Build history of the part. All positions in model axes, mm. A direction names the side the tool comes from. Coordinates: 2 decimals unless noted, no trailing zeros. Write each loop counter-clockwise with the first axis right and the second up, starting at its lowest first coordinate (ties: lowest second). Pieces come first, ordered by that corner, then holes. Notation, with made-up numbers: (-35.5, 38.5) -> (13.5, 38.5) arc R9 ccw to (13.5, 49.5) -> close; hole circle Ø3 at (15.25, 28.25). An arc over 180 degrees is marked (long way). Write each question's results on one line, items separated by ' | '. Start each with the question number.
Q1. Saw through at A-A on z = 159.5. Give the cut face in (x, y).
Q2. Drill centre lines: line 1 (X direction, y = -4.75, z = 64); line 2 (X direction, y = -1.5, z = 0) (3 decimals); line 3 (X direction, y = -3.75, z = 58). Where is each one in solid material? Low to high.
Q3. Drop flat-ended pins along their axis: pin 1 Ø2.5 at (x, z) = (-20.32, 196.85) entering from +Y; pin 2 Ø2 at (x, y) = (-15, -4.5) entering from +Z. Give the stop position or say it passes through.
Q4. Tool access for faces 1 (the face through (-15.24, -3, 54)), 2 (the face through (-17, -6.35, 107)): list every direction of +Z, -Z, +X, -X, +Y, -Y with a clear straight run to the whole face (end or side of a thin tool).
Q5. Saw through at C-C on z = 85. Give the cut face in (x, y), and give its area (3 significant figures).
Q6. Saw through at B-B on y = -1.75. Count the separate pieces of the cut face and the enclosed holes in it, and give its area (3 significant figures).
Q7. Two-plate mould, pull along Z, no slides. Class faces 3 (the face through (6.92, -3.13, 153.79)), 4 (the face through (2.115, -3.131, 195.809)), 5 (the face through (25.4, -3, 102)): released by +Z, released by -Z, zero draft, split by the parting line, or undercut.
from build123d import *

# Parameters (mm, degrees)
SKETCH1_R           = 3.96875
SKETCH1_R_2         = 15.08125
SKETCH1_R_3         = 1.5875
BOSS_EXTRUDE1_DEPTH = 6.35


with BuildPart() as part:
    # Sketch1 → Boss-Extrude1 (new body)
    with BuildSketch(Plane(origin=(0, 0, 0), x_dir=(1, 0, 0), z_dir=(0, 1, 0))):
        with BuildLine():
            Line((25.4, -39.926769414), (25.4, -166.672190904))
            ThreePointArc((25.4, -166.672190904), (25.170228885, -167.97528765), (24.508629328, -169.121211697))
            Line((24.508629328, -169.121211697), (-20.914247114, -223.254087883))
            ThreePointArc((-20.914247114, -223.254087883), (-23.728731164, -224.008226611), (-25.4, -221.621407355))
            Line((-25.4, -221.621407355), (-25.4, -39.926769414))
            ThreePointArc((-25.4, -39.926769414), (-25.169027772, -38.620377357), (-24.504115377, -37.472379149))
            add(Edge.make_bspline(
                [(-24.504115377, -37.472379149), (-15.341464403, -26.593497135), (-9.143369894, -14.104472305), (-6.985, 0)],
                knots=[0.031078099, 0.031078099, 0.031078099, 0.031078099, 1, 1, 1, 1], degree=3))
            ThreePointArc((-6.985, 0), (0, 6.985), (6.985, 0))
            add(Edge.make_bspline(
                [(24.504115377, -37.472379149), (15.363034866, -26.619107902), (9.178211427, -14.199965817), (6.985, 0)],
                knots=[0.031766068, 0.031766068, 0.031766068, 0.031766068, 1, 1, 1, 1], degree=3))
            ThreePointArc((24.504115377, -37.472379149), (25.169027772, -38.620377357), (25.4, -39.926769414))
        make_face()
        with Locations(Location((0, 0, 0), (0, 0, 270))):
            Circle(SKETCH1_R, mode=Mode.SUBTRACT)
        with Locations(Location((0, -114.3, 0), (0, 0, 270))):
            Circle(SKETCH1_R_2, mode=Mode.SUBTRACT)
        with Locations(Location((-20.32, -215.9, 0), (0, 0, 270))):
            Circle(SKETCH1_R_3, mode=Mode.SUBTRACT)
        with Locations(Location((-20.32, -209.55, 0), (0, 0, 270))):
            Circle(SKETCH1_R_3, mode=Mode.SUBTRACT)
        with Locations(Location((-20.32, -203.2, 0), (0, 0, 270))):
            Circle(SKETCH1_R_3, mode=Mode.SUBTRACT)
        with Locations(Location((-20.32, -196.85, 0), (0, 0, 270))):
            Circle(SKETCH1_R_3, mode=Mode.SUBTRACT)
        with Locations(Location((21.59, -39.926769414, 0), (0, 0, 270))):
            Circle(SKETCH1_R_3, mode=Mode.SUBTRACT)
        with BuildLine():
            Line((5.605496622, -169.473670788), (-13.166879596, -143.176324304))
            ThreePointArc((-13.166879596, -143.176324304), (-13.808086261, -142.706355865), (-14.603073846, -142.709681833))
            Line((-14.603073846, -142.709681833), (-18.395861473, -143.977201329))
            ThreePointArc((-18.395861473, -143.977201329), (-19.045805463, -144.470960171), (-19.26101006, -145.258305054))
            Line((-19.26101006, -145.258305054), (-16.771936742, -186.45833168))
            ThreePointArc((-16.771936742, -186.45833168), (-12.825939472, -191.957464848), (-6.161826947, -190.773841461))
            Line((-6.161826947, -190.773841461), (4.350250475, -181.216613261))
            ThreePointArc((4.350250475, -181.216613261), (7.209558699, -175.583695027), (5.605496622, -169.473670788))
        make_face(mode=Mode.SUBTRACT)
        with BuildLine():
            Line((4.532066161, -153.060524084), (-7.713720706, -140.184809241))
            ThreePointArc((-7.713720706, -140.184809241), (-8.755006703, -137.313107924), (-7.352336236, -134.599538218))
            ThreePointArc((-7.352336236, -134.599538218), (3.568908967, -135.592979801), (13.569379689, -131.092856661))
            ThreePointArc((13.569379689, -131.092856661), (15.024402409, -133.082319121), (14.957124713, -135.546162806))
            Line((14.957124713, -135.546162806), (8.752708503, -152.196945016))
            ThreePointArc((8.752708503, -152.196945016), (6.881732179, -153.798504677), (4.532066161, -153.060524084))
        make_face(mode=Mode.SUBTRACT)
        with BuildLine():
            Line((-12.7, -96.840386602), (-5.976567434, -78.111338504))
            ThreePointArc((-5.976567434, -78.111338504), (0, -73.906831852), (5.976567434, -78.111338504))
            Line((5.976567434, -78.111338504), (12.7, -96.840386602))
            ThreePointArc((12.7, -96.840386602), (0, -92.71), (-12.7, -96.840386602))
        make_face(mode=Mode.SUBTRACT)
        with BuildLine():
            Line((-3.370875395, -16.243299574), (-14.508125658, -37.384911468))
            ThreePointArc((-14.508125658, -37.384911468), (-15.054316585, -38.820130907), (-15.24, -40.344499969))
            Line((-15.24, -40.344499969), (-15.24, -68.284499969))
            ThreePointArc((-15.24, -68.284499969), (-12.604360524, -71.719332208), (-8.604413664, -70.062499969))
            Line((-8.604413664, -70.062499969), (-1.099852263, -57.064218334))
            ThreePointArc((-1.099852263, -57.064218334), (0, -56.429218334), (1.099852263, -57.064218334))
            Line((1.099852263, -57.064218334), (8.604413664, -70.062499969))
            ThreePointArc((8.604413664, -70.062499969), (12.604360524, -71.719332208), (15.24, -68.284499969))
            Line((15.24, -68.284499969), (15.24, -40.344499969))
            ThreePointArc((15.24, -40.344499969), (15.054316585, -38.820130907), (14.508125658, -37.384911468))
            Line((14.508125658, -37.384911468), (3.370875395, -16.243299574))
            ThreePointArc((3.370875395, -16.243299574), (0, -14.209052675), (-3.370875395, -16.243299574))
        make_face(mode=Mode.SUBTRACT)
    extrude(amount=-BOSS_EXTRUDE1_DEPTH)


solid = part.part
Returned:
1) outline: (-25.4, -6.35) -> (-18.4, -6.35) -> (-18.4, 0) -> (-25.4, 0) -> close; (-1.51, -6.35) -> (25.4, -6.35) -> (25.4, 0) -> (-1.51, 0) -> close
2) line 1: x = -25.4 to -15.24, -5.1 to 5.1, 15.24 to 25.4 | line 2: x = -6.985 to -3.969, 3.969 to 6.985 | line 3: x = -25.4 to -15.24, -1.64 to 1.64, 15.24 to 25.4
3) pin 1: passes through | pin 2: stops at z = 217.4
4) face 1: +Y, -Y | face 2: +Z, -Z, +X, -X, -Y
5) outline: (-25.4, -6.35) -> (-8.45, -6.35) -> (-8.45, 0) -> (-25.4, 0) -> close; (8.45, -6.35) -> (25.4, -6.35) -> (25.4, 0) -> (8.45, 0) -> close | area: 215 mm2
6) separate pieces: 1 | enclosed holes: 11 | area: 5,750 mm2
7) face 3: undercut | face 4: released by +Z | face 5: zero draft
